from build123d import *

# Parameters (mm, degrees)
BOSS_EXTRUDE1_DEPTH = 42
TAP1_D              = 4.134
TAP1_DEPTH          = 12.4
TAP1_TIP            = 1.2419789
TAP2_D              = 4.134
TAP2_DEPTH          = 12.4
TAP2_TIP            = 1.2419789


with BuildPart() as part:
    # Sketch1 → Boss-Extrude1 (new body)
    with BuildSketch(Plane(origin=(0, 0, 0), x_dir=(0, 0, -1), z_dir=(1, 0, 0))):
        Polygon((0, -4.618802154), (4, -2.309401077), (4, 2.309401077), (0, 4.618802154), (-4, 2.309401077), (-4, -2.309401077), align=None)
    extrude(amount=BOSS_EXTRUDE1_DEPTH)

    # Sketch2 → Cut-Revolve1 (revolve, cut)
    with BuildSketch(Plane.XY):
        Polygon((0, 4.618802154), (0.35726559, 4.618802154), (0, 4), align=None)
        Polygon((41.64273441, 4.618802154), (42, 4), (42, 4.618802154), align=None)
    revolve(axis=Axis((0, 0, 0), (1, 0, 0)), mode=Mode.SUBTRACT)

    # Tap1
    with Locations(Plane.ZY):
        with Locations((0, 0)):
            Hole(TAP1_D / 2, depth=TAP1_DEPTH)
            with Locations((0, 0, -(TAP1_DEPTH + TAP1_TIP / 2))):  # 118° drill point
                Cone(0, TAP1_D / 2, TAP1_TIP, mode=Mode.SUBTRACT)

    # Tap2
    with Locations(Plane(origin=(42, 0, 0), x_dir=(0, 0, -1), z_dir=(1, 0, 0))):
        with Locations((0, 0)):
            Hole(TAP2_D / 2, depth=TAP2_DEPTH)
            with Locations((0, 0, -(TAP2_DEPTH + TAP2_TIP / 2))):  # 118° drill point
                Cone(0, TAP2_D / 2, TAP2_TIP, mode=Mode.SUBTRACT)


solid = part.part
Can you work these out from the model? Positions are in its coordinate system, mm. A direction names the side the tool comes from. Coordinates: 2 decimals unless noted, no trailing zeros. Write each loop counter-clockwise with the first axis right and the second up, starting at its lowest first coordinate (ties: lowest second). Pieces come first, ordered by that corner, then holes.
Q1. For P1, Ø2, axis at y = 3, z = 0, coming from the -X side; P2, Ø2.5, axis at y = 0, z = 0, coming from the -X side; P3, Ø1, axis at x = 30, z = 3, coming from the +Y side, each with a flat end and sliding along its axis, tell me the tip position at first contact or that it passes through.
Results found:
P1: stops at x = 0
P2: stops at x = 12.89
P3: stops at y = 3.18
Q2. If we mould it in two halves opening along Z, with no side actions, what happens to faces 1 (the face through (21, 0, -4)), 2 (the face through (28.574, -0.35, 0.078)), 3 (the face through (41.915, -2.065, 3.597)), 4 (the face through (0.085, -4.148, 0.01))? For each: +Z half, -Z half, draft (parallel to the pull), parting line (faces both ways), or undercut.
Results found:
face 1: -Z half
face 2: undercut
face 3: +Z half
face 4: parting line
Q3. Which directions (+Z, -Z, +X, -X, +Y, -Y) give clear straight access to the entire face, cutting with the end or side of a thin tool? Please do faces 5 (the face through (0.085, -2.083, -3.587)), 6 (the face through (35.71, -1.26, -1.64)).
Results found:
face 5: -Z, -X, -Y
face 6: +X
Q4. Imagine slicing it at A-A, the plane x = 11. List the corners of the cut face in (y, z) for me.
Results found:
outline: (-4.62, 0) - (-2.31, -4) - (2.31, -4) - (4.62, 0) - (2.31, 4) - (-2.31, 4) - close; hole circle Ø4.13 at (0, 0)
Q5. Please list where these lines run through material, in increasing order: L1, parallel to Z at x = 4.25, y = 0; L2, parallel to Y at x = 3.5, z = 0; L3, parallel to Z at x = 6, y = -0.5.
Results found:
L1: z = -4 to -2.07, 2.07 to 4
L2: y = -4.62 to -2.07, 2.07 to 4.62
L3: z = -4 to -2.01, 2.01 to 4
Q6. Imagine slicing it at B-B, the plane x = 17. List the corners of the cut face in (y, z) for me.
Results found:
outline: (-4.62, 0) - (-2.31, -4) - (2.31, -4) - (4.62, 0) - (2.31, 4) - (-2.31, 4) - close
